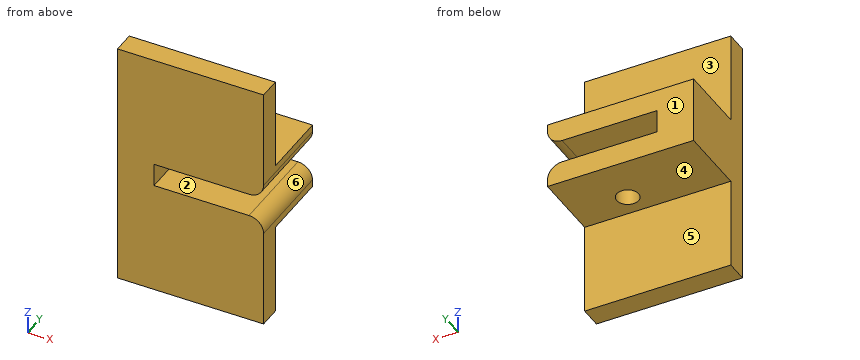
```python
from build123d import *

# Parameters (mm, degrees)
BOSS_EXTRUDE1_DEPTH = 20
SKETCH2_W           = 3.175
SKETCH2_H           = 12.5
CUT_EXTRUDE1_DEPTH  = 15
SKETCH3_R           = 1.5
CUT_EXTRUDE2_DEPTH  = 33.032103037
FILLET1_R           = 2


with BuildPart() as part:
    # Sketch1 → Boss-Extrude1 (new body)
    with BuildSketch(Plane(origin=(0, 0, 0), x_dir=(0, 0, -1), z_dir=(1, 0, 0))):
        Polygon((0, 12.5), (3, 12.5), (3, 3), (15.5, 3), (15.5, 0), (0, 0), (-3.175, 0), (-18.675, 0), (-18.675, 3), (-6.175, 3), (-6.175, 12.5), (-3.175, 12.5), align=None)
    extrude(amount=BOSS_EXTRUDE1_DEPTH)

    # Sketch2 → Cut-Extrude1 (cut)
    with BuildSketch(Plane(origin=(20, 0, 0), x_dir=(0, 0, -1), z_dir=(1, 0, 0))):
        with Locations((-1.5875, 6.25)):
            Rectangle(SKETCH2_W, SKETCH2_H)
    extrude(amount=-CUT_EXTRUDE1_DEPTH, mode=Mode.SUBTRACT)

    # Sketch3 → Cut-Extrude2 (cut, through all)
    with BuildSketch(Plane.XY.offset(6.175)):
        with Locations((12.5, 6)):
            Circle(SKETCH3_R)
    extrude(amount=-CUT_EXTRUDE2_DEPTH, mode=Mode.SUBTRACT)

    # Fillet1
    fillet1_edges = [part.edges().sort_by_distance(p)[0] for p in [
        (20, 6.25, 0),
        (20, 6.25, 3.175),
    ]]
    fillet(fillet1_edges, radius=FILLET1_R)


solid = part.part
```
Verification items for the finished model (mm, model axes). Face numbers are marked on the shaded views. A direction names the side the tool comes from. Give positions to 0.01 mm unless a question says otherwise; leave off trailing zeros. Write each loop counter-clockwise with the first axis right and the second up, starting at its lowest first coordinate (ties: lowest second). Pieces come first, ordered by that corner, then holes. Notation, with made-up numbers: (40, 1.5) - (84, 1.5) arc R18 ccw to (84, 19.5) - close; hole circle Ø5 at (63.25, 18.25). An arc over 180 degrees is marked (long way). Put each result on its own line as item: value.
Q1. Section check B-B on y = 6. Record the cut outline in (x, z) (3 decimals).
Result:
outline: (0, -3) - (11, -3) - (11, 0) - (5, 0) - (5, 3.175) - (11, 3.175) - (11, 6.175) - (0, 6.175) - close; (14, -3) - (20, -3) - (20, -2) arc R2 ccw to (18, 0) - (14, 0) - close; (14, 3.175) - (18, 3.175) arc R2 ccw to (20, 5.175) - (20, 6.175) - (14, 6.175) - close
Q2. Set-up check for the marked faces 1, 2 and 3: record each of +Z, -Z, +X, -X, +Y, -Y from which the full face is reachable in a straight line by a thin tool's end or side.
Result:
face 1: +Z, -Z, +X, -X, +Y
face 2: +X, +Y, -Y
face 3: +Z, +X, -X, +Y
Q3. Depth check by flat-ended pin: P1, Ø4, axis at x = 5, z = -10.5, coming from the +Y side; P2, Ø1, axis at y = 5, z = 1, coming from the +X side; P3, Ø4, axis at x = 13.5, y = 9, coming from the -Z side. Enter the tip coordinate at first touch or a pass-through.
Result:
P1: y = 3
P2: x = 5
P3: z = -3
Q4. Section check D-D on y = 8.75. Record the cut outline in (x, z) (3 decimals), and give its area (3 significant figures).
Result:
outline: (0, -3) - (20, -3) - (20, -2) arc R2 ccw to (18, 0) - (5, 0) - (5, 3.175) - (18, 3.175) arc R2 ccw to (20, 5.175) - (20, 6.175) - (0, 6.175) - close
area: 134 mm2
Q5. Mould release check, pull along Z, two halves, no side actions. Record for the marked faces 4, 5 and 6: released by +Z, released by -Z, zero draft, split by the parting line, or undercut.
Result:
face 4: released by -Z
face 5: zero draft
face 6: undercut
Q6. Section check A-A on x = 12.5. Record the cut outline in (y, z) (3 decimals).
Result:
outline: (0, -15.5) - (3, -15.5) - (3, -3) - (4.5, -3) - (4.5, 0) - (0, 0) - close; (0, 3.175) - (4.5, 3.175) - (4.5, 6.175) - (3, 6.175) - (3, 18.675) - (0, 18.675) - close; (7.5, -3) - (12.5, -3) - (12.5, 0) - (7.5, 0) - close; (7.5, 3.175) - (12.5, 3.175) - (12.5, 6.175) - (7.5, 6.175) - close
Q7. Section check C-C on x = 16.5. Record the cut outline in (y, z) (3 decimals), and give its area (3 significant figures).
Result:
outline: (0, -15.5) - (3, -15.5) - (3, -3) - (12.5, -3) - (12.5, 0) - (0, 0) - close; (0, 3.175) - (12.5, 3.175) - (12.5, 6.175) - (3, 6.175) - (3, 18.675) - (0, 18.675) - close
area: 150 mm2
Q8. Scan lines: probe 1 along Y at (x, z) = (12.5, -0.6); probe 2 along Z at (x, y) = (16, 1.75) (3 decimals); probe 3 along Z at (x, y) = (15.25, 11.75) (3 decimals). Record each from-to range of solid material in increasing order. Write a range as from..to.
Result:
probe 1: 0..4.5, 7.5..12.5
probe 2: -15.5..0, 3.175..18.675
probe 3: -3..0, 3.175..6.175
